from build123d import *

# Parameters (mm, degrees)
SKETCH2_R           = 1.5
BOSS_EXTRUDE1_DEPTH = 7.5
SKETCH4_W           = 8.25
SKETCH4_H           = 1.5
BOSS_EXTRUDE3_DEPTH = 20
SKETCH5_R           = 1.5
BOSS_EXTRUDE4_DEPTH = 7.5
SKETCH6_W           = 0.75
SKETCH6_H           = 0.5
CUT_EXTRUDE1_DEPTH  = 9.25
SKETCH7_R           = 1.1
CUT_EXTRUDE2_DEPTH  = 2.5
CHAMFER1_SIZE       = 1.1
FILLET1_R           = 3


with BuildPart() as part:
    # Sketch2 → Boss-Extrude1 (new body)
    with BuildSketch(Plane.XY):
        with BuildLine():
            Line((3, 3), (11.25, 3))
            Line((11.25, 3), (11.25, 1.5))
            Line((11.25, 1.5), (3, 1.5))
            Line((3, 1.5), (3, 0))
            ThreePointArc((3, 0), (0, -3), (-3, 0))
            Line((-3, 0), (-3, 2))
            Line((-3, 2), (-2.236067977, 2))
            ThreePointArc((-2.236067977, 2), (-1.224744871, 2.738612788), (0, 3))
            Line((0, 3), (3, 3))
        make_face()
        Circle(SKETCH2_R, mode=Mode.SUBTRACT)
    extrude(amount=BOSS_EXTRUDE1_DEPTH)

    # Sketch4 → Boss-Extrude3 (add)
    with BuildSketch(Plane.XY.offset(7.5)):
        with Locations((7.125, 2.25)):
            Rectangle(SKETCH4_W, SKETCH4_H)
    extrude(amount=BOSS_EXTRUDE3_DEPTH)

    # Sketch5 → Boss-Extrude4 (add)
    with BuildSketch(Plane.XY.offset(27.5)):
        with BuildLine():
            Line((11.25, 1.5), (11.25, 3))
            Line((11.25, 3), (3, 3))
            Line((3, 3), (0, 3))
            ThreePointArc((0, 3), (-1.224744871, 2.738612788), (-2.236067977, 2))
            Line((-2.236067977, 2), (-3, 2))
            Line((-3, 2), (-3, 0))
            ThreePointArc((-3, 0), (0, -3), (3, 0))
            Line((3, 0), (3, 1.5))
            Line((3, 1.5), (11.25, 1.5))
        make_face()
        Circle(SKETCH5_R, mode=Mode.SUBTRACT)
    extrude(amount=BOSS_EXTRUDE4_DEPTH)

    # Sketch6 → Cut-Extrude1 (cut, through all)
    with BuildSketch(Plane.ZY.offset(-3)):
        with Locations((19.4, 1.75)):
            Rectangle(SKETCH6_W, SKETCH6_H)
    extrude(amount=-CUT_EXTRUDE1_DEPTH, mode=Mode.SUBTRACT)

    # Sketch7 → Cut-Extrude2 (cut, through all)
    with BuildSketch(Plane.XZ.offset(-1.5)):
        with Locations((7.125, 25)):
            Circle(SKETCH7_R)
        with Locations((7.125, 10)):
            Circle(SKETCH7_R)
        with Locations((7.125, 31)):
            Circle(SKETCH7_R)
        with Locations((7.125, 4)):
            Circle(SKETCH7_R)
    extrude(amount=-CUT_EXTRUDE2_DEPTH, mode=Mode.SUBTRACT)

    # Chamfer1
    chamfer1_edges = [part.edges().sort_by_distance(p)[0] for p in [
        (6.025, 3, 4),
        (6.025, 3, 31),
        (6.025, 3, 10),
        (6.025, 3, 25),
    ]]
    chamfer(chamfer1_edges, length=CHAMFER1_SIZE)

    # Fillet1
    fillet1_edges = [part.edges().sort_by_distance(p)[0] for p in [
        (11.25, 2.25, 35),
        (11.25, 2.25, 0),
    ]]
    fillet(fillet1_edges, radius=FILLET1_R)


solid = part.part
Verification items for the finished model (mm, model axes). A direction names the side the tool comes from. Coordinates: 2 decimals unless noted, no trailing zeros. Order: outer loops, then holes, each group sorted by start corner. A loop starts at its lowest first (then second) coordinate and runs counter-clockwise, first axis right, second up.
1. Sectioned sample at A-A, the plane z = 31. Record the cut outline in (x, y) (3 decimals), and give its area (3 significant figures).
Results found:
outline: (-3, 0) arc R3 ccw to (3, 0) - (3, 1.5) - (6.025, 1.5) - (6.025, 1.9) - (4.925, 3) - (0, 3) arc R3 ccw to (-2.236, 2) - (-3, 2) - close; (8.225, 1.5) - (11.25, 1.5) - (11.25, 3) - (9.325, 3) - (8.225, 1.9) - close; hole circle Ø3 at (0, 0)
area: 31.5 mm2
2. Set-up check for faces 5 (the face through (-3, 1, 31)), 6 (the face through (7, 1.5, 27)), 7 (the face through (1.4, 1.4, 7.5)): record each of +Z, -Z, +X, -X, +Y, -Y from which the full face is reachable in a straight line by a thin tool's end or side.
Results found:
face 5: +Z, -Z, -X, +Y, -Y
face 6: +Z, -Z, +X, -Y
face 7: -X, +Y, -Y
3. Go/stop test with flat-tipped pins: pin 1 Ø0.8 at (x, z) = (-2.5, 4.5) entering from +Y; pin 2 Ø6.5 at (x, z) = (6, 11.5) entering from -Y; pin 3 Ø1 at (y, z) = (-0.5, 15.5) entering from +X; pin 4 Ø0.6 at (x, z) = (-2.5, 31.5) entering from +Y. Record where each tip stops, or that it passes through.
Results found:
pin 1: stops at y = 2.14
pin 2: stops at y = 1.5
pin 3: passes through
pin 4: stops at y = 2.04
4. Scan lines: line 1 (Z direction, x = -0.25, y = -2); line 2 (Y direction, x = 6.25, z = 20.5); line 3 (Y direction, x = 0, z = 32). Record each from-to range of solid material in increasing order.
Results found:
line 1: z = 0 to 7.5, 27.5 to 35
line 2: y = 1.5 to 3
line 3: y = -3 to -1.5, 1.5 to 3
5. Sectioned sample at B-B, the plane y = -0.5. Record the cut outline in (x, z).
Results found:
outline: (-2.96, 0) - (-1.41, 0) - (-1.41, 7.5) - (-2.96, 7.5) - close; (-2.96, 27.5) - (-1.41, 27.5) - (-1.41, 35) - (-2.96, 35) - close; (1.41, 0) - (2.96, 0) - (2.96, 7.5) - (1.41, 7.5) - close; (1.41, 27.5) - (2.96, 27.5) - (2.96, 35) - (1.41, 35) - close
6. Release check for a two-part mould opening along X. For faces 1 (the face through (6.887, 1.697, 8.926)), 2 (the face through (-1.209, 2.746, 31.197)), 3 (the face through (-1.5, 0.07, 31.2)), 4 (the face through (1.5, 0.7, 0)) record: +X half, -X half, draft (parallel to the pull), parting line (faces both ways), or undercut.
Results found:
face 1: undercut
face 2: -X half
face 3: undercut
face 4: draft
7. Sectioned sample at D-D, the plane y = 2.5. Record the cut outline in (x, z) (3 decimals).
Results found:
outline: (-1.658, 0) - (8.25, 0) arc R3 ccw to (11.25, 3) - (11.25, 32) arc R3 ccw to (8.25, 35) - (-1.658, 35) - (-1.658, 27.5) - (3, 27.5) - (3, 7.5) - (-1.658, 7.5) - close; hole circle Ø3.4 at (7.125, 4); hole circle Ø3.4 at (7.125, 10); hole circle Ø3.4 at (7.125, 25); hole circle Ø3.4 at (7.125, 31)
